```python
from build123d import *


with BuildPart() as part:
    # Sketch1 → Revolve3 (revolve)
    with BuildSketch(Plane.XY, mode=Mode.PRIVATE) as revolve3_sk:
        Polygon((0, 50), (0, 0), (50, 0), (50, 20), (4, 20), (4, 50), align=None)
        Polygon((50, 0), (0, 0), (0, -50), (4, -50), (4, -20), (50, -20), align=None)
    revolve(revolve3_sk.sketch.rotate(Axis((0, 50, 0), (0, -1, 0)), 90), axis=Axis((0, 50, 0), (0, -1, 0)))


solid = part.part
```
The model under review builds one solid part; all positions refer to its coordinate system, in mm. A direction names the side the tool comes from. Round coordinates to 2 decimals unless told otherwise and drop trailing zeros. Order: outer loops, then holes, each group sorted by start corner. A loop starts at its lowest first (then second) coordinate and runs counter-clockwise, first axis right, second up. Notation, with made-up numbers: (9.5, -22.75) - (38.5, -22.75) arc R8 cw to (38.5, -8.75) - close; hole circle Ø4 at (-9, 53). An arc over 180 degrees is marked (long way). Answer in a Markdown table with one row per item.
(1) Take a section at A-A on z = 0. Write out the cut boundary in (x, y).
Result set:
| item | result |
|---|---|
| outline | (-50, -20) - (-4, -20) - (-4, -50) - (4, -50) - (4, -20) - (50, -20) - (50, 20) - (4, 20) - (4, 50) - (-4, 50) - (-4, 20) - (-50, 20) - close |
(2) Take a section at B-B on x = 0. Write out the cut boundary in (y, z), plus the area to 3 significant figures.
Result set:
| item | result |
|---|---|
| outline | (-50, -4) - (-20, -4) - (-20, -50) - (20, -50) - (20, -4) - (50, -4) - (50, 4) - (20, 4) - (20, 50) - (-20, 50) - (-20, 4) - (-50, 4) - close |
| area | 4,480 mm2 |
(3) Take a section at D-D on y = 13.5. Write out the cut boundary in (x, z).
Result set:
| item | result |
|---|---|
| outline | circle Ø100 at (0, 0) |
(4) Mouldability with a two-part tool opening along Z and no side actions: class faces 1 (the face through (-15.02, 0.28, 47.69)), 2 (the face through (0, 50, 0)) as released by +Z, released by -Z, zero draft, split by the parting line, or undercut.
Result set:
| item | result |
|---|---|
| face 1 | split by the parting line |
| face 2 | zero draft |
(5) Take a section at C-C on y = 24. Write out the cut boundary in (x, z).
Result set:
| item | result |
|---|---|
| outline | circle Ø8 at (0, 0) |
(6) Clearance check with flat-ended pins moving along their axes: P1, Ø6, axis at y = 15.5, z = -19.5, coming from the -X side; P2, Ø10, axis at x = -24.5, z = -21, coming from the +Y side; P3, Ø5, axis at x = -0.5, y = -30, coming from the +Z side; P4, Ø12, axis at x = -10.5, y = 28, coming from the +Z side. State where each tip first meets the part, or that it passes through.
Result set:
| item | result |
|---|---|
| P1 | stops at x = -47.2 |
| P2 | stops at y = 20 |
| P3 | stops at z = 4 |
| P4 | passes through |
(7) Machinability: for faces 3 (the face through (3.905, -34.79, -0.867)), 4 (the face through (3.905, 35.21, -0.867)), 5 (the face through (0, -50, 0)), which of the approach directions +Z, -Z, +X, -X, +Y, -Y give a long, thin tool a straight path to every point of the face, cutting with its end or side? Answer none if there is none.
Result set:
| item | result |
|---|---|
| face 3 | -Y |
| face 4 | +Y |
| face 5 | +Z, -Z, +X, -X, -Y |
(8) For line 1 (Y direction, x = 28, z = 17); line 2 (Z direction, x = 8, y = 13.5); line 3 (X direction, y = 4, z = -31.5), list the stretches that pass through material, from the lowest coordinate up. Write a range as from..to.
Result set:
| item | result |
|---|---|
| line 1 | y = -20..20 |
| line 2 | z = -49.36..49.36 |
| line 3 | x = -38.83..38.83 |
